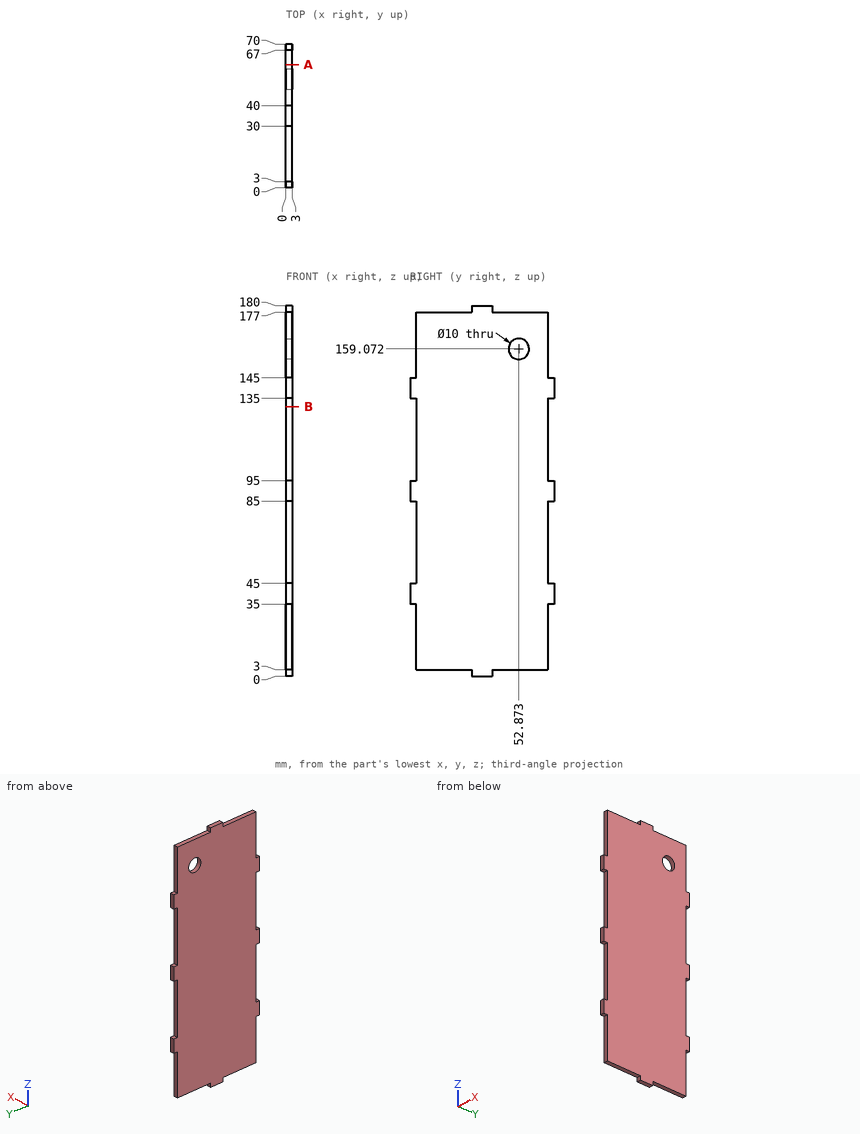
Job drawing, mm, ordinate dimensions from the low corner. One solid piece. Coordinates: 2 decimals unless noted, no trailing zeros. Order: outer loops, then holes, each group sorted by start corner. A loop starts at its lowest first (then second) coordinate and runs counter-clockwise, first axis right, second up. Notation, with made-up numbers: (82.5, 47) -> (124.5, 47) arc R26 cw to (124.5, 81) -> close; hole circle Ø4 at (-4, -10). An arc over 180 degrees is marked (long way). Answer in a Markdown table with one row per item. Add a question column.
Q1. Band-saw the part on A-A, the plane y = 60. List the corners of the cut face in (x, z), then the cut area to 3 significant figures.
Q2. Wall check: line 1 along Z through (x, y) = (2.3, 53); line 2 along Z through (x, y) = (2.2, 59); line 3 along Y through (x, z) = (1.65, 118). Give the ranges that are in metal, low to high. Write a range as [from, to].
Q3. Drop flat-ended pins along their axis: pin 1 (0.9 mm diameter, centred on x = 2, y = 68.5, fed in from +Z); pin 2 (1.5 mm diameter, centred on x = 1.5, z = 59.5, fed in from -Y); pin 3 (1.5 mm diameter, centred on x = 2, z = 179, fed in from -Y). Give the stop position or say it passes through.
Q4. Band-saw the part on B-B, the plane z = 131. List the corners of the cut face in (x, y), then the cut area to 3 significant figures.
Answers follow:
| question | item | result |
|---|---|---|
| 1 | outline | (0, 3) -> (3, 3) -> (3, 177) -> (0, 177) -> close |
| 1 | area | 522 mm^2 |
| 2 | line 1 | [3, 154.07], [164.07, 177] |
| 2 | line 2 | [3, 177] |
| 2 | line 3 | [3, 67] |
| 3 | pin 1 | z = 145 |
| 3 | pin 2 | y = 3 |
| 3 | pin 3 | y = 30 |
| 4 | outline | (0, 3) -> (3, 3) -> (3, 67) -> (0, 67) -> close |
| 4 | area | 192 mm^2 |
